```python
from build123d import *

# Parameters (mm, degrees)
SKETCH1_W             = 177.8
SKETCH1_H             = 114.3
SKETCH1_W_2           = 165.1
SKETCH1_H_2           = 16.134929366
BOSS_EXTRUDE1_DEPTH   = 4.7625
CUT_EXTRUDE1_DEPTH    = 5.7625
SKETCH4_R             = 2.38125
CUT_EXTRUDE2_DEPTH    = 5.7625
F_6_32_TAPPED_HOLE1_D = 2.7051
SKETCH7_W             = 12.7
SKETCH7_H             = 4.7625
BOSS_EXTRUDE2_DEPTH   = 4.7625
SKETCH8_W             = 12.7
SKETCH8_H             = 4.7625
BOSS_EXTRUDE3_DEPTH   = 4.7625


with BuildPart() as part:
    # Sketch1 → Boss-Extrude1 (new body)
    with BuildSketch(Plane(origin=(0, 0, 0), x_dir=(1, 0, 0), z_dir=(0, 1, 0))):
        Rectangle(SKETCH1_W, SKETCH1_H)
        with BuildLine():
            Line((-82.55, -25.4), (-82.55, -20.767464683))
            Line((-82.55, -20.767464683), (82.55, -20.767464683))
            Line((82.55, -20.767464683), (82.55, -25.4))
            ThreePointArc((82.55, -25.4), (64.589487758, -32.839487758), (57.15, -50.8))
            Line((57.15, -50.8), (-57.15, -50.8))
            ThreePointArc((-57.15, -50.8), (-64.589487758, -32.839487758), (-82.55, -25.4))
        make_face(mode=Mode.SUBTRACT)
        Rectangle(SKETCH1_W_2, SKETCH1_H_2, mode=Mode.SUBTRACT)
        with BuildLine():
            Line((82.55, 20.767464683), (-82.55, 20.767464683))
            Line((-82.55, 20.767464683), (-82.55, 25.4))
            ThreePointArc((-82.55, 25.4), (-64.589487758, 32.839487758), (-57.15, 50.8))
            Line((-57.15, 50.8), (57.15, 50.8))
            ThreePointArc((57.15, 50.8), (64.589487758, 32.839487758), (82.55, 25.4))
            Line((82.55, 25.4), (82.55, 20.767464683))
        make_face(mode=Mode.SUBTRACT)
    extrude(amount=BOSS_EXTRUDE1_DEPTH)

    # Sketch3 → Cut-Extrude1 (cut, through all)
    with BuildSketch(Plane(origin=(0, 4.7625, 0), x_dir=(1, 0, 0), z_dir=(0, 1, 0))):
        with BuildLine():
            Line((-73.406, 16.004964683), (73.406, 16.004964683))
            ThreePointArc((73.406, 16.004964683), (74.9935, 14.417464683), (73.406, 12.829964683))
            Line((73.406, 12.829964683), (-73.406, 12.829964683))
            ThreePointArc((-73.406, 12.829964683), (-74.9935, 14.417464683), (-73.406, 16.004964683))
        make_face()
        with BuildLine():
            Line((-73.406, -16.004964683), (73.406, -16.004964683))
            ThreePointArc((73.406, -16.004964683), (74.9935, -14.417464683), (73.406, -12.829964683))
            Line((73.406, -12.829964683), (-73.406, -12.829964683))
            ThreePointArc((-73.406, -12.829964683), (-74.9935, -14.417464683), (-73.406, -16.004964683))
        make_face()
    extrude(amount=-CUT_EXTRUDE1_DEPTH, mode=Mode.SUBTRACT)

    # Sketch4 → Cut-Extrude2 (cut, through all)
    with BuildSketch(Plane(origin=(0, 4.7625, 0), x_dir=(1, 0, 0), z_dir=(0, 1, 0))):
        with Locations((-73.406, 39.37)):
            Circle(SKETCH4_R)
        with Locations((-73.406, -39.37)):
            Circle(SKETCH4_R)
        with Locations((73.406, -39.37)):
            Circle(SKETCH4_R)
        with Locations((73.406, 39.37)):
            Circle(SKETCH4_R)
    extrude(amount=-CUT_EXTRUDE2_DEPTH, mode=Mode.SUBTRACT)

    # #6-32 Tapped Hole1 (through all)
    with Locations(Plane(origin=(0, 6.2865, 0), x_dir=(-1, 0, 0), z_dir=(0, 1, 0))):
        with Locations((82.55, -50.8), (82.55, 50.8), (-82.55, 50.8), (-82.55, -50.8)):
            Hole(F_6_32_TAPPED_HOLE1_D / 2)

    # Sketch7 → Boss-Extrude2 (add)
    with BuildSketch(Plane.ZY.offset(88.9)):
        with Locations((-12.7, 2.38125)):
            Rectangle(SKETCH7_W, SKETCH7_H)
        with Locations((38.1, 2.38125)):
            Rectangle(SKETCH7_W, SKETCH7_H)
    extrude(amount=BOSS_EXTRUDE2_DEPTH)

    # Sketch8 → Boss-Extrude3 (add)
    with BuildSketch(Plane(origin=(88.9, 0, 0), x_dir=(0, 0, -1), z_dir=(1, 0, 0))):
        with Locations((-12.7, 2.38125)):
            Rectangle(SKETCH8_W, SKETCH8_H)
        with Locations((38.1, 2.38125)):
            Rectangle(SKETCH8_W, SKETCH8_H)
    extrude(amount=BOSS_EXTRUDE3_DEPTH)


solid = part.part
```
Source: CAD feature listing. Evaluate the final solid. Frame: model axes, mm. A direction names the side the tool comes from. Round coordinates to 2 decimals unless told otherwise and drop trailing zeros. Loops run counter-clockwise (first coordinate to the right, second up) from the corner with the lowest first, then second, coordinate; pieces in that order, holes last. Notation, with made-up numbers: M -28.75,-24 L -1.75,-24 A24 ccw -1.75,9 Z; hole C -5,77 d4. An arc over 180 degrees is marked long. Use a Markdown table: item, result. Add a question column.
1. Mould query, pull axis X, two halves, no side actions, for faces 4 (the flat face through (-88.9, 2, 51)), 5 (the flat face through (-1, 2, -16.005)), 6 (the flat face through (-91, 2, -6.35)). Classes: pulls with the +X half, pulls with the -X half, needs draft (parallel to the pull), parting line crosses it, or undercut.
2. Section query A-A on x = -5.5. Return the cut outline in (y, z), then the cut area to 3 significant figures.
3. Section query B-B on z = -29. Return the cut outline in (x, y).
4. Contact query for flat-ended pins moving along their axis: P1, Ø2.5, axis at y = 3, z = 23.5, coming from the -X side; P2, Ø2.5, axis at x = -91.5, y = 2.5, coming from the -Z side; P3, Ø2, axis at x = 82.55, z = 50.8, coming from the +Y side; P4, Ø2.5, axis at y = 2.5, z = -2.5, coming from the +X side. Output: stop coordinate, or through.
5. Section query C-C on z = 39.37. Return the cut outline in (x, y), then the cut area to 3 significant figures.
6. Line query: line 1 (Z direction, x = -4, y = 0.8); line 2 (X direction, y = 4.1, z = 6); line 3 (Z direction, x = -61, y = 1.05). Output: solid intervals per line, ascending.
7. Reachability of faces 1 (the flat face through (82.55, 2, 0)), 2 (the flat face through (88.9, 2, -12)), 3 (the flat face through (91, 2, -44.45)) from +Z, -Z, +X, -X, +Y, -Y: full face, straight path, thin tool, end or side. Return the list, or none.
8. Section query D-D on y = 1.1. Give the number of separate pieces and of enclosed holes in the cut face, then the cut area to 3 significant figures.
Reported:
| question | item | result |
|---|---|---|
| 1 | face 4 | pulls with the -X half |
| 1 | face 5 | undercut |
| 1 | face 6 | needs draft |
| 2 | outline | M 0,-57.15 L 4.76,-57.15 L 4.76,-50.8 L 0,-50.8 Z; M 0,-20.77 L 4.76,-20.77 L 4.76,-16 L 0,-16 Z; M 0,-12.83 L 4.76,-12.83 L 4.76,-8.07 L 0,-8.07 Z; M 0,8.07 L 4.76,8.07 L 4.76,12.83 L 0,12.83 Z; M 0,16 L 4.76,16 L 4.76,20.77 L 0,20.77 Z; M 0,50.8 L 4.76,50.8 L 4.76,57.15 L 0,57.15 Z |
| 2 | area | 151 mm² |
| 3 | outline | M -88.9,0 L -69.51,0 L -69.51,4.76 L -88.9,4.76 Z; M 69.51,0 L 88.9,0 L 88.9,4.76 L 69.51,4.76 Z |
| 4 | P1 | stops at x = -88.9 |
| 4 | P2 | stops at z = -19.05 |
| 4 | P3 | passes through |
| 4 | P4 | stops at x = 88.9 |
| 5 | outline | M -93.66,0 L -75.79,0 L -75.79,4.76 L -93.66,4.76 Z; M -71.02,0 L -59.87,0 L -59.87,4.76 L -71.02,4.76 Z; M 59.87,0 L 71.02,0 L 71.02,4.76 L 59.87,4.76 Z; M 75.79,0 L 88.9,0 L 88.9,4.76 L 75.79,4.76 Z |
| 5 | area | 254 mm² |
| 6 | line 1 | z = -57.15 to -50.8, -20.77 to -16, -12.83 to -8.07, 8.07 to 12.83, 16 to 20.77, 50.8 to 57.15 |
| 6 | line 2 | x = -88.9 to -82.55, 82.55 to 88.9 |
| 6 | line 3 | z = -57.15 to -37.36, -20.77 to -16, -12.83 to -8.07, 8.07 to 12.83, 16 to 20.77, 37.36 to 57.15 |
| 7 | face 1 | +Y, -Y |
| 7 | face 2 | +X, +Y, -Y |
| 7 | face 3 | -Z, +X, +Y, -Y |
| 8 | separate pieces | 1 |
| 8 | enclosed holes | 13 |
| 8 | area | 8,970 mm² |
